Input: part model. Units: mm. Frame: model coordinates. A direction names the side the tool comes from. Coordinates: 2 decimals unless noted, no trailing zeros. Loops run counter-clockwise (first coordinate to the right, second up) from the corner with the lowest first, then second, coordinate; pieces in that order, holes last.
```python
from build123d import *

# Parameters (mm, degrees)
SKETCH1_R             = 5
BOSS_EXTRUDE1_DEPTH   = 0.1
BOSS_EXTRUDE1_2_DEPTH = 0.1
BOSS_EXTRUDE1_3_DEPTH = 0.1
BOSS_EXTRUDE1_4_DEPTH = 0.1
BOSS_EXTRUDE2_DEPTH   = 3
SKETCH3_R             = 3
CUT_EXTRUDE1_DEPTH    = 3


with BuildPart() as part:
    # Sketch1 → Boss-Extrude1 (new body)
    with BuildSketch(Plane.XY):
        with Locations((-44.491847198, 44.491847198)):
            Circle(SKETCH1_R)
    extrude(amount=BOSS_EXTRUDE1_DEPTH)



with BuildPart() as body_2:
    # Sketch1 → Boss-Extrude1 2 (new body)
    with BuildSketch(Plane.XY):
        with Locations((44.491847198, 44.491847198)):
            Circle(SKETCH1_R)
    extrude(amount=BOSS_EXTRUDE1_2_DEPTH)


with BuildPart() as body_3:
    # Sketch1 → Boss-Extrude1 3 (new body)
    with BuildSketch(Plane.XY):
        with Locations((44.491847198, -44.491847198)):
            Circle(SKETCH1_R)
    extrude(amount=BOSS_EXTRUDE1_3_DEPTH)


with BuildPart() as body_4:
    # Sketch1 → Boss-Extrude1 4 (new body)
    with BuildSketch(Plane.XY):
        with Locations((-44.491847198, -44.491847198)):
            Circle(SKETCH1_R)
    extrude(amount=BOSS_EXTRUDE1_4_DEPTH)


with BuildPart() as part_1:
    add(part.part)

    add(body_2.part)  # Boss-Extrude2 merges body 2

    add(body_3.part)  # Boss-Extrude2 merges body 3

    add(body_4.part)  # Boss-Extrude2 merges body 4
    # Sketch2 → Boss-Extrude2 (add)
    with BuildSketch(Plane.XY):
        with BuildLine():
            Line((-59.341089603, 40.956313292), (-40.956313292, 59.341089603))
            ThreePointArc((-40.956313292, 59.341089603), (0, 73.058676231), (40.956313292, 59.341089603))
            Line((40.956313292, 59.341089603), (59.341089603, 40.956313292))
            ThreePointArc((59.341089603, 40.956313292), (39.686643359, 0), (59.341089603, -40.956313292))
            Line((59.341089603, -40.956313292), (40.956313292, -59.341089603))
            ThreePointArc((40.956313292, -59.341089603), (0, -73.058676231), (-40.956313292, -59.341089603))
            Line((-40.956313292, -59.341089603), (-59.341089603, -40.956313292))
            ThreePointArc((-59.341089603, -40.956313292), (-39.686643359, 0), (-59.341089603, 40.956313292))
        make_face()
        with BuildLine():
            Line((-38.750824491, 48.750824491), (0, 10))
            Line((0, 10), (38.750824491, 48.750824491))
            ThreePointArc((38.750824491, 48.750824491), (0, 64.323437718), (-38.750824491, 48.750824491))
        make_face(mode=Mode.SUBTRACT)
        with BuildLine():
            Line((-37.410135101, 29.495739933), (-10, 0))
            Line((-10, 0), (-37.410135101, -29.495739933))
            ThreePointArc((-37.410135101, -29.495739933), (-38.724006049, -29.628666123), (-39.024062115, -28.342628566))
            ThreePointArc((-39.024062115, -28.342628566), (-31.907853639, 0), (-39.024062115, 28.342628566))
            ThreePointArc((-39.024062115, 28.342628566), (-38.724006049, 29.628666123), (-37.410135101, 29.495739933))
        make_face(mode=Mode.SUBTRACT)
        with BuildLine():
            Line((10, 0), (37.410135101, -29.495739933))
            ThreePointArc((37.410135101, -29.495739933), (38.724006049, -29.628666123), (39.024062115, -28.342628566))
            ThreePointArc((39.024062115, -28.342628566), (31.907853639, 0), (39.024062115, 28.342628566))
            ThreePointArc((39.024062115, 28.342628566), (38.724006049, 29.628666123), (37.410135101, 29.495739933))
            Line((37.410135101, 29.495739933), (10, 0))
        make_face(mode=Mode.SUBTRACT)
        with BuildLine():
            Line((0, -10), (38.750824491, -48.750824491))
            ThreePointArc((38.750824491, -48.750824491), (0, -64.323437718), (-38.750824491, -48.750824491))
            Line((-38.750824491, -48.750824491), (0, -10))
        make_face(mode=Mode.SUBTRACT)
    extrude(amount=BOSS_EXTRUDE2_DEPTH)

    # Sketch3 → Cut-Extrude1 (cut)
    with BuildSketch(Plane.XY.offset(3)):
        with Locations((-44.5, -41.5)):
            Circle(SKETCH3_R)
        with Locations((44.5, -41.5)):
            Circle(SKETCH3_R)
        with Locations((44.5, 41.5)):
            Circle(SKETCH3_R)
        with Locations((-44.5, 41.5)):
            Circle(SKETCH3_R)
    extrude(amount=-CUT_EXTRUDE1_DEPTH, mode=Mode.SUBTRACT)


solid = part_1.part
```
Item 1: Contact query for a flat-ended pin moving along its axis: P1, Ø1.5, axis at x = -30.5, z = 1, coming from the +Y side. Output: stop coordinate, or through.
Result:
P1: stops at y = 66.21
Item 2: Reachability of faces 4 (the face through (39.69, 0.66, 1.48)), 5 (the face through (-31.91, -0.41, 1.48)) from +Z, -Z, +X, -X, +Y, -Y: full face, straight path, thin tool, end or side. Return the list, or none.
Result:
face 4: +Z, -Z, +X
face 5: +Z, -Z
Item 3: Line query: L1, parallel to Y at x = 0, z = 0.7; L2, parallel to Y at x = -0.5, z = 2; L3, parallel to Y at x = 20.5, z = 0.95 (3 decimals). Output: solid intervals per line, ascending.
Result:
L1: y = -73.06 to -64.32, -10 to 10, 64.32 to 73.06
L2: y = -73.06 to -64.32, -10.5 to 10.5, 64.32 to 73.06
L3: y = -69.895 to -60.436, -30.5 to -11.299, 11.299 to 30.5, 60.436 to 69.895
Item 4: Section query D-D (x = 35). Output: boundary loops of the cut face in (y, z).
Result:
outline: (-63.36, 0) - (-52.04, 0) - (-52.04, 3) - (-63.36, 3) - close; (-45, 0) - (-26.9, 0) - (-26.9, 3) - (-45, 3) - close; (-19.01, 0) - (19.01, 0) - (19.01, 3) - (-19.01, 3) - close; (26.9, 0) - (45, 0) - (45, 3) - (26.9, 3) - close; (52.04, 0) - (63.36, 0) - (63.36, 3) - (52.04, 3) - close
Item 5: Section query C-C (z = 2.55). Count the separate pieces of the cut face and the enclosed holes in it, then the cut area to 3 significant figures.
Result:
separate pieces: 1
enclosed holes: 8
area: 6,660 mm2
Item 6: Section query A-A (x = -19). Output: boundary loops of the cut face in (y, z), then the cut area to 3 significant figures.
Result:
outline: (-70.35, 0) - (-61, 0) - (-61, 3) - (-70.35, 3) - close; (-29, 0) - (-9.68, 0) - (-9.68, 3) - (-29, 3) - close; (9.68, 0) - (29, 0) - (29, 3) - (9.68, 3) - close; (61, 0) - (70.35, 0) - (70.35, 3) - (61, 3) - close
area: 172 mm2
Item 7: Mould query, pull axis Y, two halves, no side actions, for faces 1 (the face through (-0.615, 73.056, 1.479)), 2 (the face through (31.91, -0.41, 1.48)), 3 (the face through (1, 1, 0)). Classes: +Y half, -Y half, draft (parallel to the pull), parting line (faces both ways), or undercut.
Result:
face 1: +Y half
face 2: undercut
face 3: draft
Item 8: Section query B-B (y = 22.5). Output: boundary loops of the cut face in (x, z), then the cut area to 3 significant figures.
Result:
outline: (-44.75, 0) - (-36.29, 0) - (-36.29, 3) - (-44.75, 3) - close; (-30.91, 0) - (-12.5, 0) - (-12.5, 3) - (-30.91, 3) - close; (12.5, 0) - (30.91, 0) - (30.91, 3) - (12.5, 3) - close; (36.29, 0) - (44.75, 0) - (44.75, 3) - (36.29, 3) - close
area: 161 mm2
